Source: three-view drawing plus pictorial views. Frame: mm from the lowest corner of the part. A direction names the side the tool comes from. Give positions to 0.01 mm unless a question says otherwise; leave off trailing zeros. Loops run counter-clockwise (first coordinate to the right, second up) from the corner with the lowest first, then second, coordinate; pieces in that order, holes last. Notation, with made-up numbers: M 46,38 L 57,38 A23 cw 57,71 Z; hole C -6.75,-30.5 d1. An arc over 180 degrees is marked long. Answer as a JSON object with one key per item and string values. Group by question number.
1) First-contact query: P1, Ø7.5, axis at x = 37.5, y = 13, coming from the +Z side; P2, Ø12, axis at x = 51.5, y = 14.5, coming from the -Z side; P3, Ø5, axis at x = 14, z = 54.5, coming from the +Y side (1 decimal); P4, Ø8, axis at y = 12, z = 50.5, coming from the -X side. Flat tips, straight axial feed; report the tip coordinate or a pass-through.
2) Section query D-D on x = 38.5. Return loops of the section in (y, z).
3) Access query for the marked faces 1 and 2. Directions: +Z, -Z, +X, -X, +Y, -Y. A direction counts if a zero-diameter tool reaches every point of the face in a straight line with its end or side. Return the directions, or none.
4) Section query C-C on z = 63.5. Return loops of the section in (x, y).
5) Section query B-B on x = 11. Return loops of the section in (y, z), plus the area to 3 significant figures.
6) Section query A-A on y = 17.5. Return loops of the section in (x, z).
7) Ray query, L1, parallel to Z at x = 50.5, y = 2; L2, parallel to X at y = 16, z = 49; L3, parallel to X at y = 15.5, z = 43. Return the intervals inside material, ascending.
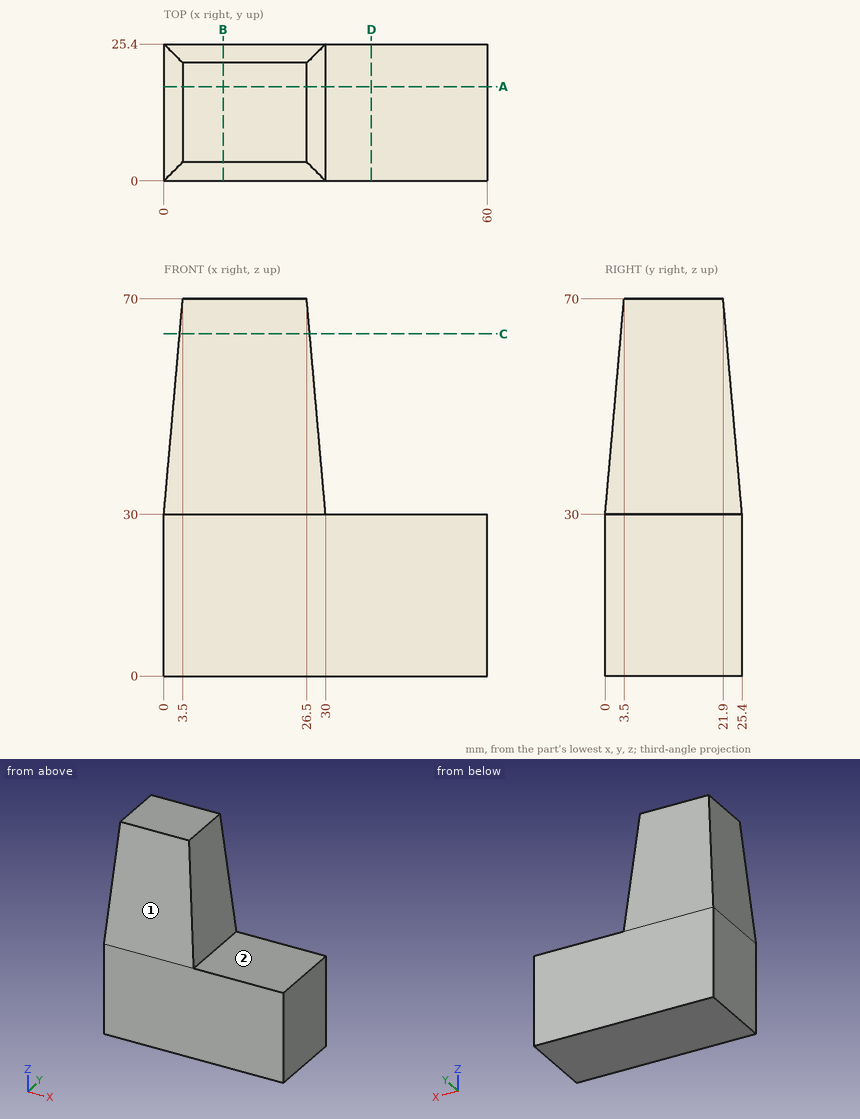
Output:
{
 "1": {"P1": "stops at z = 30", "P2": "stops at z = 0", "P3": "stops at y = 23.5", "P4": "stops at x = 1.44"},
 "2": {"outline": "M 0,0 L 25.4,0 L 25.4,30 L 0,30 Z"},
 "3": {"face 1": "+Z, +X, -X, -Y", "face 2": "+Z, +X, +Y, -Y"},
 "4": {"outline": "M 2.93,2.93 L 27.07,2.93 L 27.07,22.47 L 2.93,22.47 Z"},
 "5": {"outline": "M 0,0 L 25.4,0 L 25.4,30 L 21.9,70 L 3.5,70 L 0,30 Z", "area": "1,640 mm^2"},
 "6": {"outline": "M 0,0 L 60,0 L 60,30 L 30,30 L 26.5,70 L 3.5,70 L 0,30 Z"},
 "7": {"L1": "z = 0 to 30", "L2": "x = 1.66 to 28.34", "L3": "x = 1.14 to 28.86"}
}
